Geometry check sheet. Reference: the model listing, model coordinates, mm. Face numbers are marked on the shaded views. A direction names the side the tool comes from. Give positions to 0.01 mm unless a question says otherwise; leave off trailing zeros. Write each loop counter-clockwise with the first axis right and the second up, starting at its lowest first coordinate (ties: lowest second). Pieces come first, ordered by that corner, then holes. Notation, with made-up numbers: (51.25, -38.75) -> (68.25, -38.75) arc R12 ccw to (68.25, -26.75) -> close; hole circle Ø4 at (5.5, 28). An arc over 180 degrees is marked (long way). Use a Markdown table: item, result. Add a question column.
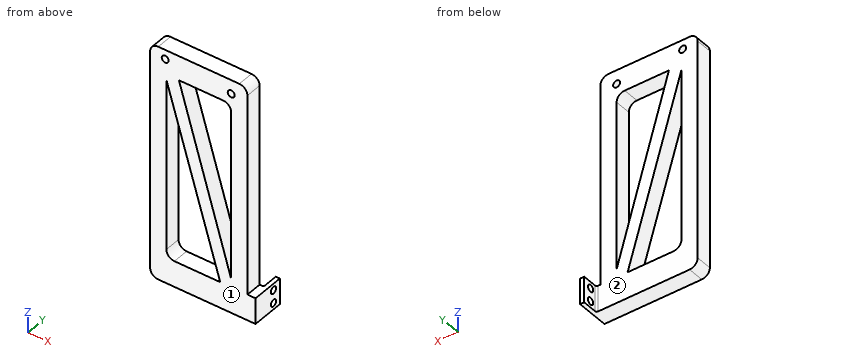
from build123d import *

# Parameters (mm, degrees)
EXTRUDE_1_DEPTH     = 10
SKETCH_4_W          = 2.5
SKETCH_4_H          = 16
EXTRUDE_2_DEPTH     = 10
CUT_EXTRUDE_1_REACH = 103.606
SKETCH_5_R          = 2.15
CUT_EXTRUDE_2_REACH = 93.602
SKETCH_6_R          = 2.15
FILLET_1_R          = 5
FILLET_2_R          = 5
FILLET_3_R          = 1


with BuildPart() as part:
    # 草图1 → 凸台-拉伸1 (new body)
    with BuildSketch(Plane(origin=(0, 0, 0), x_dir=(1, 0, 0), z_dir=(0, 1, 0))):
        Polygon((0.431150433, 77.572237736), (47.680774799, 77.572237736), (47.680774799, 61.572237736), (42.680774799, 61.572237736), (42.680774799, 31.757290204), (42.680774799, -57.600660719), (42.680774799, -67.427762264), (0.431150433, -67.427762264), (-17.319225201, -67.427762264), (-17.319225201, 77.572237736), align=None)
        Polygon((25.906315323, 61.572237736), (-7.319225201, 61.572237736), (-7.319225201, -49.220735683), align=None, mode=Mode.SUBTRACT)
        Polygon((0.431150433, -52.427762264), (32.680774799, -52.427762264), (32.680774799, 56.508121895), align=None, mode=Mode.SUBTRACT)
    extrude(amount=EXTRUDE_1_DEPTH)

    # 草图4 → 凸台-拉伸2 (add)
    with BuildSketch(Plane(origin=(0, 10, 0), x_dir=(1, 0, 0), z_dir=(0, 1, 0))):
        with Locations((46.430774799, 69.572237736)):
            Rectangle(SKETCH_4_W, SKETCH_4_H)
    extrude(amount=EXTRUDE_2_DEPTH)

    # 草图5 → 切除-拉伸1 (cut, up to next)
    with BuildSketch(Plane.ZY.offset(-45.180774799), mode=Mode.PRIVATE) as cut_extrude_1_sk1:
        with Locations((-73.607625165, 14.752522231)):
            Circle(SKETCH_5_R)
    cut_extrude_1_tool1 = extrude(cut_extrude_1_sk1.sketch, amount=-CUT_EXTRUDE_1_REACH, mode=Mode.PRIVATE) & part.part
    # 草图5 → 切除-拉伸1 (cut, up to next)
    with BuildSketch(Plane.ZY.offset(-45.180774799), mode=Mode.PRIVATE) as cut_extrude_1_sk2:
        with Locations((-65.607625165, 14.752522231)):
            Circle(SKETCH_5_R)
    cut_extrude_1_tool2 = extrude(cut_extrude_1_sk2.sketch, amount=-CUT_EXTRUDE_1_REACH, mode=Mode.PRIVATE) & part.part
    add(cut_extrude_1_tool1.solids().sort_by_distance((45.180775, 14.752522, -73.607625))[0], mode=Mode.SUBTRACT)
    add(cut_extrude_1_tool2.solids().sort_by_distance((45.180775, 14.752522, -65.607625))[0], mode=Mode.SUBTRACT)

    # 草图6 → 切除-拉伸2 (cut, up to next)
    with BuildSketch(Plane(origin=(0, 10, 0), x_dir=(1, 0, 0), z_dir=(0, 1, 0)), mode=Mode.PRIVATE) as cut_extrude_2_sk1:
        with Locations(Location((-8.019225201, -61.690086649, 0), (0, 0, 270))):
            Circle(SKETCH_6_R)
    cut_extrude_2_tool1 = extrude(cut_extrude_2_sk1.sketch, amount=-CUT_EXTRUDE_2_REACH, mode=Mode.PRIVATE) & part.part
    # 草图6 → 切除-拉伸2 (cut, up to next)
    with BuildSketch(Plane(origin=(0, 10, 0), x_dir=(1, 0, 0), z_dir=(0, 1, 0)), mode=Mode.PRIVATE) as cut_extrude_2_sk2:
        with Locations(Location((32.680774799, -58.840086649, 0), (0, 0, 270))):
            Circle(SKETCH_6_R)
    cut_extrude_2_tool2 = extrude(cut_extrude_2_sk2.sketch, amount=-CUT_EXTRUDE_2_REACH, mode=Mode.PRIVATE) & part.part
    add(cut_extrude_2_tool1.solids().sort_by_distance((-8.019225, 10, 61.690087))[0], mode=Mode.SUBTRACT)
    add(cut_extrude_2_tool2.solids().sort_by_distance((32.680775, 10, 58.840087))[0], mode=Mode.SUBTRACT)

    # 圆角1
    fillet_1_edges = [part.edges().sort_by_distance(p)[0] for p in [
        (-17.319225201, 5, 67.427762264),
        (-17.319225201, 5, -77.572237736),
        (42.680774799, 5, 67.427762264),
    ]]
    fillet(fillet_1_edges, radius=FILLET_1_R)

    # 圆角2
    fillet_2_edges = [part.edges().sort_by_distance(p)[0] for p in [
        (-7.319225201, 5, -61.572237736),
        (32.680774799, 5, 52.427762264),
    ]]
    fillet(fillet_2_edges, radius=FILLET_2_R)

    # 圆角3
    fillet_3_edges = [part.edges().sort_by_distance(p)[0] for p in [
        (45.180774799, 10, -69.572237736),
    ]]
    fillet(fillet_3_edges, radius=FILLET_3_R)


solid = part.part
1) Sectioned sample at A-A, the plane x = 14.5. Enter the section's corners in (y, z).
2) Sectioned sample at B-B, the plane z = -4.5. Enter the section's corners in (x, y).
3) Tool access check on the marked faces 1 and 2. Record the directions out of +Z, -Z, +X, -X, +Y, -Y that give a thin tool (end or side, any length) a straight path to the whole face; none if there is none.
4) Material ranges on probe 1 along X at (y, z) = (3.5, 36); probe 2 along X at (y, z) = (2.75, 16.5); probe 3 along Z at (x, y) = (-8, 4), recorded low to high. Write a range as [from, to].
5) Sectioned sample at D-D, the plane x = -4. Enter the section's corners in (y, z).
6) Sectioned sample at C-C, the plane y = 6. Enter the section's corners in (x, z), and give its area (3 significant figures).
7) Gauge pin test, flat ends, axial feed: P1, Ø11, axis at y = 7, z = 0, coming from the +X side; P2, Ø10, axis at y = 13.5, z = -70, coming from the -X side; P3, Ø1, axis at x = -8.5, z = 27, coming from the +Y side. Record the tip position at first contact, or that the pin passes through.
Check values:
| question | item | result |
|---|---|---|
| 1 | outline | (0, -77.57) -> (10, -77.57) -> (10, -61.57) -> (0, -61.57) -> close; (0, -23.54) -> (10, -23.54) -> (10, 4.9) -> (0, 4.9) -> close; (0, 52.43) -> (10, 52.43) -> (10, 67.43) -> (0, 67.43) -> close |
| 2 | outline | (-17.32, 0) -> (-7.32, 0) -> (-7.32, 10) -> (-17.32, 10) -> close; (8.79, 0) -> (17.28, 0) -> (17.28, 10) -> (8.79, 10) -> close; (32.68, 0) -> (42.68, 0) -> (42.68, 10) -> (32.68, 10) -> close |
| 3 | face 1 | +Z, -Z, +X, -X, -Y |
| 3 | face 2 | +Z, -Z, -X, +Y |
| 4 | probe 1 | [-17.32, -7.32], [-3.35, 5.29], [32.68, 42.68] |
| 4 | probe 2 | [-17.32, -7.32], [2.49, 11.07], [32.68, 42.68] |
| 4 | probe 3 | [-77.57, 59.54], [63.84, 67.43] |
| 5 | outline | (0, -77.57) -> (10, -77.57) -> (10, -61.28) -> (0, -61.28) -> close; (0, 38.15) -> (10, 38.15) -> (10, 67.43) -> (0, 67.43) -> close |
| 6 | outline | (-17.32, -72.57) arc R5 ccw to (-12.32, -77.57) -> (47.68, -77.57) -> (47.68, -61.57) -> (42.68, -61.57) -> (42.68, 62.43) arc R5 ccw to (37.68, 67.43) -> (-12.32, 67.43) arc R5 ccw to (-17.32, 62.43) -> close; hole circle Ø4.3 at (-8.02, 61.69); hole (-7.32, -56.57) arc R5 ccw to (-2.32, -61.57) -> (25.91, -61.57) -> (-7.32, 49.22) -> close; hole (0.43, 52.43) -> (32.68, -56.51) -> (32.68, 47.43) arc R5 ccw to (27.68, 52.43) -> close; hole circle Ø4.3 at (32.68, 58.84) |
| 6 | area | 5,150 mm² |
| 7 | P1 | x = 42.68 |
| 7 | P2 | x = -17.32 |
| 7 | P3 | y = 10 |
